Read the model definition and answer for the solid it produces. Units are mm, in the model's axes. Face numbers are marked on the shaded views. Round coordinates to 2 decimals unless told otherwise and drop trailing zeros. Loops run counter-clockwise (first coordinate to the right, second up) from the corner with the lowest first, then second, coordinate; pieces in that order, holes last. Notation, with made-up numbers: (1.25, -28) - (5.25, -28) arc R14 cw to (5.25, -9) - close; hole circle Ø2 at (-3, -6). An arc over 180 degrees is marked (long way). Use CSV: the item, a comma, the result in double quotes. Start each with the question number.
1. Find section C-C (x = 1.75). Give the vertices of the cut face in (y, z).
2. Find section D-D (x = 8.5). Give the vertices of the cut face in (y, z).
3. Determine the mould class of the marked faces 1, 2, 3 and 4 for opening direction X: +X half, -X half, draft (parallel to the pull), parting line (faces both ways), or undercut.
4. Find section B-B (z = -4). Give the vertices of the cut face in (x, y), and give its area (3 significant figures).
5. Given pin 1 Ø9 at (x, y) = (0, 0) entering from -Z; pin 2 Ø1 at (x, z) = (-5, -6) entering from -Y, each flat-ended and moving along its own axis, determine where each tip first touches the part or whether it passes through.
6. Consider line 1 along Y through (x, z) = (0, -3.75); line 2 along Y through (x, z) = (1, -1.5); line 3 along X through (y, z) = (-0.5, -2.25). Determine where each line is inside the solid, lowest interval first.
7. Find section A-A (x = -4). Give the vertices of the cut face in (y, z), and give its area (3 significant figures).
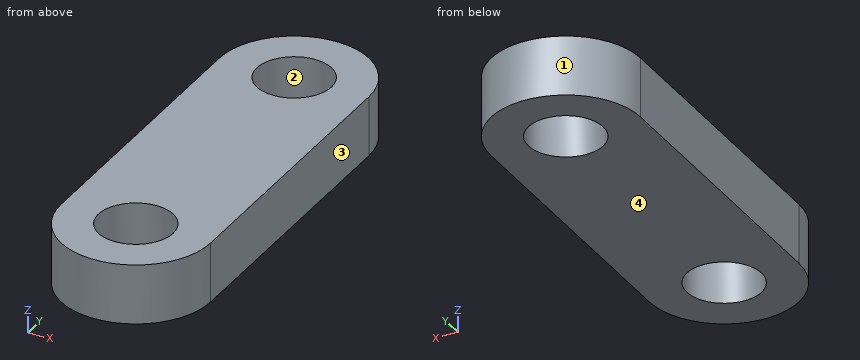
from build123d import *

# Parameters (mm, degrees)
SKETCH1_R           = 5
BOSS_EXTRUDE1_DEPTH = 8


with BuildPart() as part:
    # Sketch1 → Boss-Extrude1 (new body)
    with BuildSketch(Plane.XY):
        with BuildLine():
            Line((10, 0), (10, 40))
            ThreePointArc((10, 40), (0, 50), (-10, 40))
            Line((-10, 40), (-10, 0))
            ThreePointArc((-10, 0), (0, -10), (10, 0))
        make_face()
        with Locations((0, 40)):
            Circle(SKETCH1_R, mode=Mode.SUBTRACT)
        Circle(SKETCH1_R, mode=Mode.SUBTRACT)
    extrude(amount=-BOSS_EXTRUDE1_DEPTH)


solid = part.part
Filled sheet:
1,outline,"(-9.85, -8) - (-4.68, -8) - (-4.68, 0) - (-9.85, 0) - close; (4.68, -8) - (35.32, -8) - (35.32, 0) - (4.68, 0) - close; (44.68, -8) - (49.85, -8) - (49.85, 0) - (44.68, 0) - close"
2,outline,"(-5.27, -8) - (45.27, -8) - (45.27, 0) - (-5.27, 0) - close"
3,face 1,"parting line"
3,face 2,"undercut"
3,face 3,"+X half"
3,face 4,"draft"
4,outline,"(-10, 0) arc R10 ccw to (10, 0) - (10, 40) arc R10 ccw to (-10, 40) - close; hole circle Ø10 at (0, 0); hole circle Ø10 at (0, 40)"
4,area,"957 mm²"
5,pin 1,"passes through"
5,pin 2,"stops at y = -8.93"
6,line 1,"y = -10 to -5, 5 to 35, 45 to 50"
6,line 2,"y = -9.95 to -4.9, 4.9 to 35.1, 44.9 to 49.95"
6,line 3,"x = -9.99 to -4.97, 4.97 to 9.99"
7,outline,"(-9.17, -8) - (-3, -8) - (-3, 0) - (-9.17, 0) - close; (3, -8) - (37, -8) - (37, 0) - (3, 0) - close; (43, -8) - (49.17, -8) - (49.17, 0) - (43, 0) - close"
7,area,"371 mm²"
